Autodesk Inventor part; units mm, degrees
ref_plane "YZ Plane" through (0, 0, 0) normal (1, 0, 0) x (0, 1, 0)
ref_plane "XZ Plane" through (0, 0, 0) normal (0, 1, 0) x (-1, 0, 0)
ref_plane "XY Plane" through (0, 0, 0) normal (0, 0, 1) x (1, 0, 0)
sketch "Sketch1" plane through (0, 0, 0) normal (0, 0, 1) x (1, 0, 0)
  line L0 (0, 20) -> (0, 0)
  line L1 (0, 0) -> (50, 8.8163)
  line L2 (0, 20) -> (-3, 20)
  line L3 (-3, 20) -> (-3, -4.5907)
  line L4 (-3, -4.5907) -> (50.6946, 4.8771)
  line L5 (0, 0) -> (50.6946, 0) construction
  line L6 (50, 8.8163) -> (50.6946, 4.8771)
  line L7 (0, 20) -> (50, 20)
  line L8 (50, 20) -> (50, 8.8163)
  line L9 (50.3473, 6.8467) -> (11.5175, 0) construction
  dimension "d0" = 20
  dimension "d1" = 3
  dimension "d2" = 10
  dimension "d3" = 4
  dimension "d4" = 50
extrude "Plate1" add sketch "Sketch1" along normal mid plane 3
fillet "Corner Round1" radius 2 1 edges at (50, 8.8163, 0)
equation "\"d5\" = Thickness"
equation "\"BendRadius\" = Thickness"
equation "\"BendReliefWidth\" = Thickness"
equation "\"BendReliefDepth\" = 0.5 * Thickness"
equation "\"CornerReliefSize\" = 4 * Thickness"
equation "\"MinimumRemnant\" = 2 * Thickness"
equation "\"TransitionRadius\" = BendRadius"
equation "\"JacobiRadiusSize\" = BendRadius"
equation "\"GapSize\" = Thickness"
properties part number "Ramp Side Wall"
Geometry: final body of the model. Coordinates: model frame, mm. A direction names the side the tool comes from. Give positions to 0.01 mm unless a question says otherwise; leave off trailing zeros. Loops run counter-clockwise (first coordinate to the right, second up) from the corner with the lowest first, then second, coordinate; pieces in that order, holes last. Notation, with made-up numbers: (20, -26) -> (35, -26) arc R31 ccw to (35, 3) -> close; hole circle Ø11 at (74.5, 2). An arc over 180 degrees is marked (long way). Use one line per item in the form item = value.
Item 1: Section query B-B on x = 17.5. Output: boundary loops of the cut face in (y, z).
A:
outline = (-0.98, -1.5) -> (20, -1.5) -> (20, 1.5) -> (-0.98, 1.5) -> close
Item 2: Section query C-C on y = 0.5. Output: boundary loops of the cut face in (x, z).
A:
outline = (-3, -1.5) -> (25.87, -1.5) -> (25.87, 1.5) -> (-3, 1.5) -> close
Item 3: Line query: probe 1 along X at (y, z) = (18, -0.6); probe 2 along Y at (x, z) = (1, 0.7); probe 3 along Y at (x, z) = (31, 0.85). Output: solid intervals per line, ascending.
A:
probe_1 = -3 to 50
probe_2 = -3.89 to 20
probe_3 = 1.4 to 20
Item 4: Access query for faces 1 (the face through (50, 15, 0)), 2 (the face through (23, 11, -1.5)). Directions: +Z, -Z, +X, -X, +Y, -Y. A direction counts if a zero-diameter tool reaches every point of the face in a straight line with its end or side. Return the directions, or none.
A:
face_1 = +Z, -Z, +X, +Y
face_2 = -Z, +X, -X, +Y, -Y
Item 5: Section query A-A on z = 0.4. Output: boundary loops of the cut face in (x, y), and give its area (3 significant figures).
A:
outline = (-3, -4.59) -> (50.69, 4.88) -> (50.03, 8.64) arc R2 cw to (50, 8.99) -> (50, 20) -> (-3, 20) -> close
area = 1,060 mm^2
